The model under review builds one solid part; all positions refer to its coordinate system, in mm. Coordinates: 2 decimals unless noted, no trailing zeros.
from build123d import *

# Parameters (mm, degrees)
EXTRUDE_1_DEPTH          = 5
FILLET_6_R               = 5
FILLET_7_R               = 2
FILLET_8_R               = 5
CUT_EXTRUDE_1_DEPTH      = 185.424559073
CUT_EXTRUDE_1_DEPTH_BACK = 185.424559073
SKETCH_6_W               = 27.094284284
SKETCH_6_H               = 20.392851323
CUT_EXTRUDE_2_DEPTH      = 164.712248904
SKETCH_7_W               = 91.771448639
SKETCH_7_H               = 20.028601632
CUT_EXTRUDE_3_DEPTH      = 167.349688769


# Read off the part's stored shape, not the designer's step: 凸台-拉伸1
with BuildPart() as part:
    # 凸台-拉伸1 outline → 凸台-拉伸1 (new body)
    with BuildSketch(Plane(origin=(0, 0, 0), x_dir=(0, 0, -1), z_dir=(1, 0, 0))):
        with BuildLine():
            add(Edge.make_bspline(
                [(0, -14.903846424), (2.951295662, -4.14849373), (13.496276672, -1.883966721), (29.52909514, 0), (83.401333812, 0)],
                knots=[0, 0, 0, 0, 0, 1, 1, 1, 1, 1], degree=4))
            add(Edge.make_bspline(
                [(0, -14.903846424), (13.738939295, -26.332723654), (29.4774768, -32.710998586), (74.674999713, -39.156033076), (130, -39.931386408)],
                knots=[0, 0, 0, 0, 0, 0.958214361, 0.958214361, 0.958214361, 0.958214361, 0.958214361], degree=4))
            Line((130, -39.931386408), (130, -20))
            add(Edge.make_bspline(
                [(130, -20), (142.554964398, -11.053747082), (149.196912904, -34.934175524), (158.630756241, -5.373255264), (163.289648635, -33.936740498), (166.072200522, -10.144868391), (180, -20)],
                knots=[0, 0, 0, 0, 0, 0, 0, 1, 1, 1, 1, 1, 1, 1], degree=6))
            Line((180, -20), (180, 0))
            Line((180, 0), (83.401333812, 0))
        make_face()
    extrude(amount=EXTRUDE_1_DEPTH)

    # 圆角6
    fillet_6_edges = [part.edges().sort_by_distance(p)[0] for p in [
        (2.5, -20, -130),
    ]]
    fillet(fillet_6_edges, radius=FILLET_6_R)

    # 圆角7
    fillet_7_edges = [part.edges().sort_by_distance(p)[0] for p in [
        (2.5, -20, -180),
    ]]
    fillet(fillet_7_edges, radius=FILLET_7_R)

    # 圆角8
    fillet_8_edges = [part.edges().sort_by_distance(p)[0] for p in [
        (2.5, 0, -180),
        (2.5, -39.931386408, -130),
    ]]
    fillet(fillet_8_edges, radius=FILLET_8_R)

    # 草图4 → 切除-拉伸1 (cut, two sides: drawn at the far end of the back side and taken through both)
    with BuildSketch(Plane(origin=(5, 0, 0), x_dir=(0, 0, -1), z_dir=(1, 0, 0)).offset(-CUT_EXTRUDE_1_DEPTH_BACK)):
        with BuildLine():
            add(Edge.make_bspline(
                [(1.495142471, -11.305529877), (14.835007519, -23.95714683), (75.592167753, -33.882807925), (104.343520452, -34.842413885), (130, -34.842413885)],
                knots=[0, 0, 0, 0, 0, 1, 1, 1, 1, 1], degree=4))
            add(Edge.make_bspline(
                [(0, -14.903846424), (0.275551051, -13.899660779), (0.617298034, -12.969491649), (1.023527011, -12.106738133), (1.495142471, -11.305529877)],
                knots=[0, 0, 0, 0, 0, 0.093366129, 0.093366129, 0.093366129, 0.093366129, 0.093366129], degree=4))
            add(Edge.make_bspline(
                [(0, -14.903846424), (13.419828476, -26.067268054), (28.7474456, -32.411980768), (71.57295957, -38.706985512), (124.893658481, -39.841282905)],
                knots=[0, 0, 0, 0, 0, 0.935958162, 0.935958162, 0.935958162, 0.935958162, 0.935958162], degree=4))
            add(Edge.make_bspline(
                [(130, -34.842413884), (130, -35.028759319), (129.99166601, -35.216258569), (129.974804907, -35.404332472), (129.94928895, -35.592386619), (129.915057389, -35.77981586), (129.841480351, -36.098859681), (129.806409214, -36.231082745), (129.766907364, -36.362456276), (129.722994517, -36.492760695), (129.674707397, -36.621778563), (129.58487848, -36.839515421), (129.545494286, -36.928984789), (129.503966151, -37.017626664), (129.46031708, -37.10536636), (129.414574093, -37.192130532), (129.250587102, -37.486161652), (129.122218575, -37.688294916), (128.98211374, -37.883204904), (128.830848248, -38.069925037), (128.669117931, -38.247570978), (128.255836276, -38.652154349), (127.994673555, -38.869333518), (127.716552177, -39.064613196), (127.424118002, -39.236250049), (127.120264983, -39.382959218), (126.679539096, -39.553907949), (126.549523427, -39.599440156), (126.418314531, -39.640571717), (126.286130578, -39.677270539), (126.153191519, -39.709521582), (125.832655006, -39.776296457), (125.644540113, -39.806533973), (125.455985822, -39.828044566), (125.267595854, -39.840901842), (125.079961766, -39.845246156), (124.893658481, -39.841282905)],
                knots=[0, 0, 0, 0, 0, 0, 0, 0.145130031, 0.145130031, 0.145130031, 0.145130031, 0.145130031, 0.248682026, 0.248682026, 0.248682026, 0.248682026, 0.248682026, 0.321947701, 0.321947701, 0.321947701, 0.321947701, 0.321947701, 0.500002972, 0.500002972, 0.500002972, 0.500002972, 0.500002972, 0.751317975, 0.751317975, 0.751317975, 0.751317975, 0.751317975, 0.85486997, 0.85486997, 0.85486997, 0.85486997, 0.85486997, 1, 1, 1, 1, 1, 1, 1], degree=6))
        make_face()
    extrude(amount=CUT_EXTRUDE_1_DEPTH + CUT_EXTRUDE_1_DEPTH_BACK, mode=Mode.SUBTRACT)

    # 草图6 → 切除-拉伸2 (cut, through all)
    with BuildSketch(Plane(origin=(57.793484303, -9.892917122, -28.873774023), x_dir=(-0.4401729492006857, 0.04581450966450186, -0.8967434446351822), z_dir=(0.88426202268349, -0.1513653487033851, -0.4417795903520281))):
        with Locations((120.420599257, -28.887536231)):
            Rectangle(SKETCH_6_W, SKETCH_6_H)
    extrude(amount=CUT_EXTRUDE_2_DEPTH, mode=Mode.SUBTRACT)

    # 草图7 → 切除-拉伸3 (cut, through all)
    with BuildSketch(Plane(origin=(-53.53520172, -9.024374029, -26.444544598), x_dir=(-0.43181481098590574, -0.07279057966413091, 0.8990203003966966), z_dir=(-0.886513170069574, -0.14943861555354754, -0.437906952987314))):
        with Locations((-105.176126902, -32.909539251)):
            Rectangle(SKETCH_7_W, SKETCH_7_H)
    extrude(amount=CUT_EXTRUDE_3_DEPTH, mode=Mode.SUBTRACT)


solid = part.part
(1) Insertion check: pin 1 Ø1.5 at (x, y) = (1, -7.5) entering from +Z. The pin has a flat end and moves straight along its axis. Give the tip position at first contact, or say it passes through.
(2) The part is to be moulded in two halves that separate along X. For faces 1 (the face through (4.305, -31.591, -128.502)), 2 (the face through (0, -13, -92)), 3 (the face through (2, -28, -130)), say which applies: +X half, -X half, draft (parallel to the pull), parting line (faces both ways), or undercut.
(3) Wall thickness on line 1 (Y direction, x = 0.6, z = -104); line 2 (Z direction, x = 0.3, y = -9.5); line 3 (Z direction, x = 2.35, y = -12): over which ranges is each line inside the solid? List them lowest first.
Findings:
1. pin 1: stops at z = -3.99
2. face 1: +X half
2. face 2: -X half
2. face 3: draft
3. line 1: y = -34.17 to 0
3. line 2: z = -180 to -2.78
3. line 3: z = -180 to -2.28
